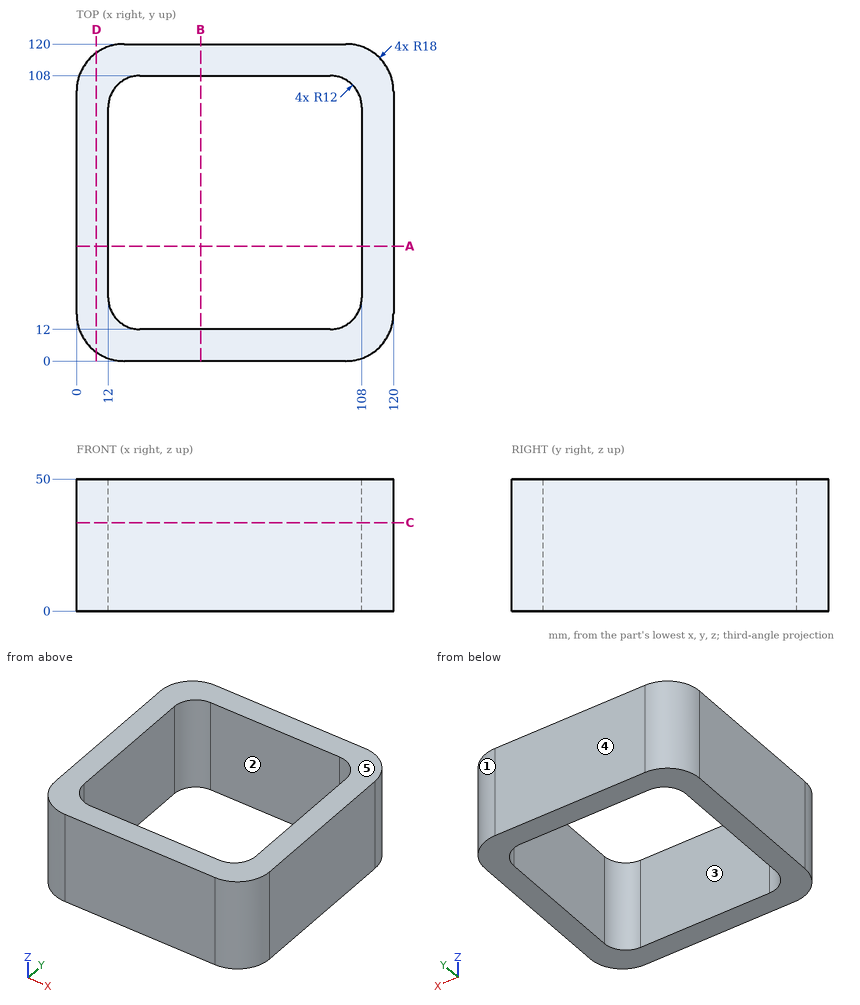
Geometry check sheet. Reference: drawing and pictorial views, mm from the part's lowest x, y, z. A direction names the side the tool comes from. Round coordinates to 2 decimals unless told otherwise and drop trailing zeros. Loops run counter-clockwise (first coordinate to the right, second up) from the corner with the lowest first, then second, coordinate; pieces in that order, holes last.
1. Set-up check for the marked faces 1 and 2: record each of +Z, -Z, +X, -X, +Y, -Y from which the full face is reachable in a straight line by a thin tool's end or side.
2. Sectioned sample at C-C on z = 33.5. Record the boundary of the cut face in (x, y).
3. Sectioned sample at A-A on y = 43.5. Record the boundary of the cut face in (x, z), and give its area (3 significant figures).
4. Sectioned sample at D-D on x = 7.5. Record the boundary of the cut face in (y, z).
5. Mould release check, pull along Y, two halves, no side actions. Record for the marked faces 3, 4 and 5: released by +Y, released by -Y, zero draft, split by the parting line, or undercut.
6. Scan lines: probe 1 along Y at (x, z) = (74.5, 11.5); probe 2 along X at (y, z) = (96.5, 28); probe 3 along Y at (x, z) = (19, 3). Record each from-to range of solid material in increasing order.
7. Gauge pin test, flat end, axial feed: pin 1 Ø3 at (x, z) = (105, 27.5) entering from +Y. Record the tip position at first contact, or that the pin passes through.
Recorded:
1. face 1: +Z, -Z, +X, +Y
1. face 2: +Z, -Z
2. outline: (0, 18) arc R18 ccw to (18, 0) - (102, 0) arc R18 ccw to (120, 18) - (120, 102) arc R18 ccw to (102, 120) - (18, 120) arc R18 ccw to (0, 102) - close; hole (12, 24) arc R12 ccw to (24, 12) - (96, 12) arc R12 ccw to (108, 24) - (108, 96) arc R12 ccw to (96, 108) - (24, 108) arc R12 ccw to (12, 96) - close
3. outline: (0, 0) - (12, 0) - (12, 50) - (0, 50) - close; (108, 0) - (120, 0) - (120, 50) - (108, 50) - close
3. area: 1,200 mm2
4. outline: (3.38, 0) - (116.62, 0) - (116.62, 50) - (3.38, 50) - close
5. face 3: undercut
5. face 4: released by +Y
5. face 5: zero draft
6. probe 1: y = 0 to 12, 108 to 120
6. probe 2: x = 0 to 12.01, 107.99 to 120
6. probe 3: y = 0 to 13.09, 106.91 to 120
7. pin 1: stops at y = 119.94
